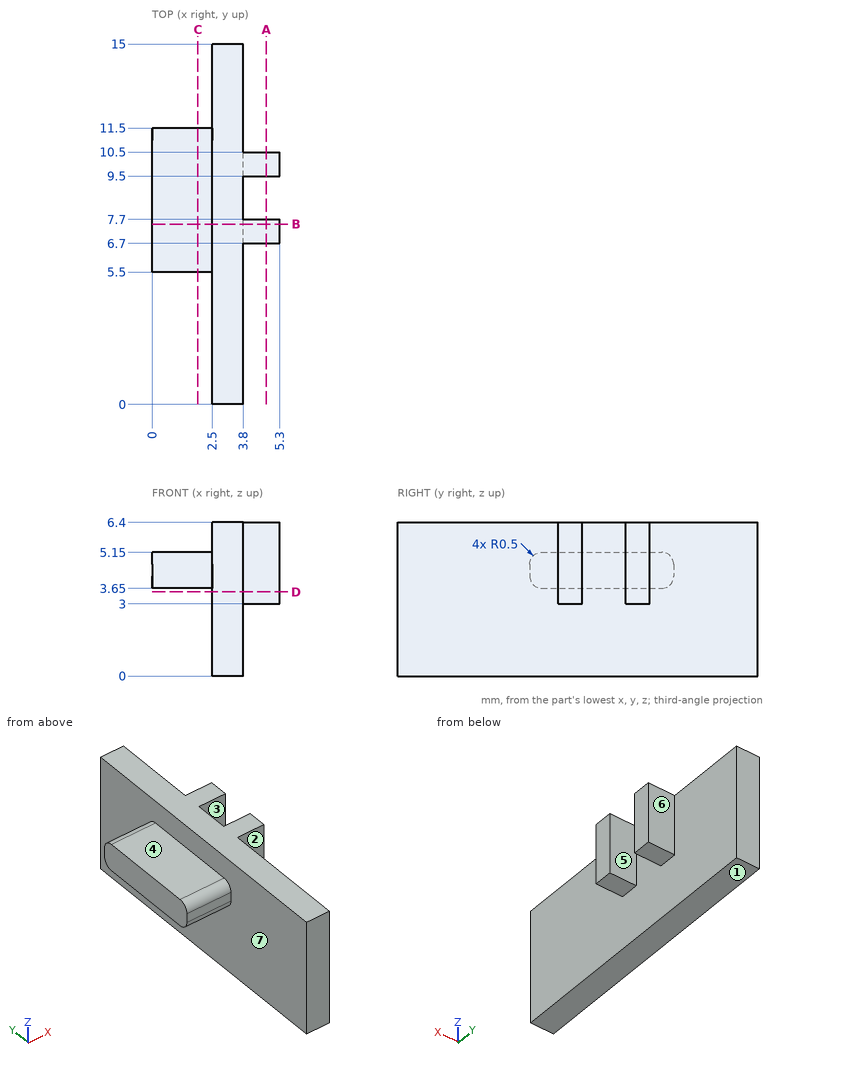
Geometry check sheet. Reference: drawing and pictorial views, mm from the part's lowest x, y, z. A direction names the side the tool comes from. Coordinates: 2 decimals unless noted, no trailing zeros. Loops run counter-clockwise (first coordinate to the right, second up) from the corner with the lowest first, then second, coordinate; pieces in that order, holes last. Notation, with made-up numbers: (73.5, -2) - (101.5, -2) arc R19 ccw to (101.5, 4) - close; hole circle Ø10 at (9.25, 85.25). An arc over 180 degrees is marked (long way). Return JSON: item names as keys, results as strings.
1. Section check B-B, the plane y = 7.5. Record the boundary of the cut face in (x, z).
Established:
{"outline": "(0, 3.65) - (2.5, 3.65) - (2.5, 0) - (3.8, 0) - (3.8, 3) - (5.3, 3) - (5.3, 6.4) - (2.5, 6.4) - (2.5, 5.15) - (0, 5.15) - close"}
2. Mould release check, pull along Y, two halves, no side actions. Record for the marked faces 5, 6 and 7: +Y half, -Y half, draft (parallel to the pull), parting line (faces both ways), or undercut.
Established:
{"face 5": "undercut", "face 6": "+Y half", "face 7": "draft"}
3. Section check C-C, the plane x = 1.9. Record the boundary of the cut face in (y, z), then the cut area to 3 significant figures.
Established:
{"outline": "(5.5, 4.15) arc R0.5 ccw to (6, 3.65) - (11, 3.65) arc R0.5 ccw to (11.5, 4.15) - (11.5, 4.65) arc R0.5 ccw to (11, 5.15) - (6, 5.15) arc R0.5 ccw to (5.5, 4.65) - close", "area": "8.79 mm2"}
4. Thickness scan on L1, parallel to Y at x = 4.1, z = 3.75; L2, parallel to X at y = 5.25, z = 6; L3, parallel to Z at x = 0.95, y = 8. Record the ranges inside material, lowest first.
Established:
{"L1": "y = 6.7 to 7.7, 9.5 to 10.5", "L2": "x = 2.5 to 3.8", "L3": "z = 3.65 to 5.15"}
5. Section check D-D, the plane z = 3.5. Record the boundary of the cut face in (x, y), then the cut area to 3 significant figures.
Established:
{"outline": "(2.5, 0) - (3.8, 0) - (3.8, 6.7) - (5.3, 6.7) - (5.3, 7.7) - (3.8, 7.7) - (3.8, 9.5) - (5.3, 9.5) - (5.3, 10.5) - (3.8, 10.5) - (3.8, 15) - (2.5, 15) - close", "area": "22.5 mm2"}
6. Tool access check on the marked faces 1, 2, 3 and 4. Record the directions out of +Z, -Z, +X, -X, +Y, -Y that give a thin tool (end or side, any length) a straight path to the whole face; none if there is none.
Established:
{"face 1": "-Z, +X, -X, +Y, -Y", "face 2": "+Z, -Z, +X, -Y", "face 3": "+Z, -Z, +X", "face 4": "+Z, -X, +Y, -Y"}
7. Section check A-A, the plane x = 4.75. Record the boundary of the cut face in (y, z), then the cut area to 3 significant figures.
Established:
{"outline": "(6.7, 3) - (7.7, 3) - (7.7, 6.4) - (6.7, 6.4) - close; (9.5, 3) - (10.5, 3) - (10.5, 6.4) - (9.5, 6.4) - close", "area": "6.80 mm2"}
8. Go/stop test with flat-tipped pins: pin 1 (0.5 mm diameter, centred on x = 5, y = 7, fed in from -Z); pin 2 (0.6 mm diameter, centred on x = 1.5, z = 4.5, fed in from +Y); pin 3 (1.2 mm diameter, centred on x = 4.5, z = 5, fed in from +Y). Record where each tip stops, or that it passes through.
Established:
{"pin 1": "stops at z = 3", "pin 2": "stops at y = 11.5", "pin 3": "stops at y = 10.5"}
